from build123d import *


# Read off the part's stored shape, not the designer's step: M12 机械螺纹 螺柱1
with BuildPart() as part:
    # 草图1 → 旋转1 (revolve)
    with BuildSketch(Plane.XY, mode=Mode.PRIVATE) as revolve_1_sk:
        with BuildLine():
            Line((60, 0), (60, 6))
            Line((60, 6), (7, 6))
            ThreePointArc((7, 6), (5.585786438, 6.585786438), (5, 8))
            Line((5, 8), (5, 9))
            Line((5, 9), (0, 9))
            ThreePointArc((0, 9), (-1.597221966, 4.625396092), (-2.139428901, 0))
            Line((-2.139428901, 0), (60, 0))
        make_face()
    revolve(revolve_1_sk.sketch.rotate(Axis((0, 0, 0), (1, 0, 0)), 90), axis=Axis((0, 0, 0), (1, 0, 0)))

    # M12 机械螺纹 螺柱1 outline → M12 机械螺纹 螺柱1 (revolve, cut)
    with BuildSketch(Plane.YX):
        Polygon((6, 60), (5.053, 60), (6, 59.053), align=None)
    revolve(axis=Axis((0, 0, 0), (1, 0, 0)), mode=Mode.SUBTRACT)


solid = part.part
Geometry check sheet. Reference: the model listing, model coordinates, mm. A direction names the side the tool comes from. Round coordinates to 2 decimals unless told otherwise and drop trailing zeros. Order: outer loops, then holes, each group sorted by start corner. A loop starts at its lowest first (then second) coordinate and runs counter-clockwise, first axis right, second up. Notation, with made-up numbers: (5, 36.5) - (16, 36.5) arc R25 cw to (16, 73.5) - close; hole circle Ø2 at (70.25, 22.5). An arc over 180 degrees is marked (long way). One line per question, with ' | ' between items. Start each with the question number.
(1) Thickness scan on L1, parallel to Y at x = 26, z = 3.25; L2, parallel to Z at x = 33.5, y = 0.25. Record the ranges inside material, lowest first. Write a range as [from, to].
(2) Sectioned sample at C-C on x = 54.5. Record the cut outline in (y, z).
(3) Access from +Z, -Z, +X, -X, +Y, -Y to the whole of each face (thin tool, end or side, straight path). Record for faces 1 (the cylindrical face through (2.465, -6.083, -6.633)), 2 (the cylindrical face through (32.662, -1.802, 5.723)).
(4) Sectioned sample at A-A on z = 0. Record the cut outline in (x, y), and give its area (3 significant figures).
(5) Depth check by flat-ended pin: pin 1 Ø1 at (y, z) = (4, -4) entering from -X; pin 2 Ø2 at (x, z) = (36.5, -3.5) entering from +Y; pin 3 Ø5 at (y, z) = (0.5, 5.5) entering from -X. Enter the tip coordinate at first touch or a pass-through.
Conclusion:
1) L1: y = [-5.04, 5.04] | L2: z = [-5.99, 5.99]
2) outline: circle Ø12 at (0, 0)
3) face 1: +X, -X | face 2: +X
4) outline: (0, -9) - (5, -9) - (5, -8) arc R2 cw to (7, -6) - (59.05, -6) - (60, -5.05) - (60, 5.05) - (59.05, 6) - (7, 6) arc R2 cw to (5, 8) - (5, 9) - (0, 9) arc R20 ccw to start | area: 777 mm2
5) pin 1: stops at x = -1.46 | pin 2: stops at y = 5.45 | pin 3: stops at x = -1.91
